Read the model definition and answer for the solid it produces. Units are mm, in the model's axes. A direction names the side the tool comes from. Coordinates: 2 decimals unless noted, no trailing zeros. Order: outer loops, then holes, each group sorted by start corner. A loop starts at its lowest first (then second) coordinate and runs counter-clockwise, first axis right, second up. Notation, with made-up numbers: M 10,59 L 16,59 A19 cw 16,93 Z; hole C 34.5,22 d11. An arc over 180 degrees is marked long. Use a Markdown table: item, result. Add a question column.
1) Find section B-B on y = 10. Write down the section's boundary in (x, z).
2) The mould has two halves that part along X. Classify faces 3 (the face through (1.012, 8.874, 15.317)), 4 (the face through (20.99, 0.493, 16.094)), 5 (the face through (-11, 0, -11)): released by +X, released by -X, zero draft, split by the parting line, or undercut.
3) For faces 1 (the face through (-5, 3, -20)), 2 (the face through (10.15, 1.479, 17.756)), determine the directions among +Z, -Z, +X, -X, +Y, -Y from which every point of the face is accessible in a straight line to the end or side of a thin tool.
4) Find section C-C on y = 4. Write down the section's boundary in (x, z), plus the area to 3 significant figures.
5) Find the intervals of material crossed by probe 1 along Z at (x, y) = (0, 8.75); probe 2 along Y at (x, z) = (22, 7.5); probe 3 along Z at (x, y) = (-22.45, 0.85), in increasing order. Write a range as [from, to].
6) Each of these flat-tipped pins is pushed along its axis until it touches: pin 1 Ø10 at (x, y) = (5.5, 14.5) entering from -Z; pin 2 Ø3.5 at (x, z) = (11.22, -19.44) entering from +Y (3 decimals); pin 3 Ø2 at (y, z) = (10, -1.5) entering from -X; pin 4 Ø5 at (x, z) = (11.22, 19.44) entering from +Y. Where does it stop, or does it pass through?
Autodesk Inventor part; units mm, degrees
ref_plane "YZ Plane" through (0, 0, 0) normal (1, 0, 0) x (0, 1, 0)
ref_plane "XZ Plane" through (0, 0, 0) normal (0, 1, 0) x (-1, 0, 0)
ref_plane "XY Plane" through (0, 0, 0) normal (0, 0, 1) x (1, 0, 0)
sketch "Sketch1" plane through (0, 0, 0) normal (0, 1, 0) x (-1, 0, 0)
  circle A0 centre (0, 0) radius 26.45
  circle A1 centre (22.45, 0) radius 2
  circle A2 centre (0, 0) radius 22.45 construction
  circle A3 centre (-11.225, 19.4423) radius 2
  circle A4 centre (-11.225, -19.4423) radius 2
  circle A5 centre (0, 0) radius 15.35
  dimension "d0" = 52.9
  dimension "d1" = 4
  dimension "d2" = 4
  dimension "d5" = 360
  dimension "d7" = 30.7
extrude "Extrusion1" add sketch "Sketch1" along normal blind 3
sketch "Sketch2" plane through (0, 3, 0) normal (0, 1, 0) x (1, 0, 0)
  circle A0 centre (0, 0) radius 15.35
  circle A1 centre (11.225, 19.4423) radius 2
  circle A2 centre (11.225, -19.4423) radius 2
  circle A3 centre (-22.45, 0) radius 2
  circle A4 centre (0, 0) radius 26.45
  circle A5 centre (0, 0) radius 18.35
  dimension "d10" = 3
extrude "Extrusion2" add sketch "Sketch2" along normal blind 15 contours A5
fillet "Fillet1" radius 2 2 edges at (-18.35, 3, 0) (26.45, 3, 0)
properties part number "00_Zeiss_eyepieceport"
Check result:
| question | item | result |
|---|---|---|
| 1 | outline | C 0,0 d36.7; hole C 0,0 d30.7 |
| 2 | face 3 | undercut |
| 2 | face 4 | split by the parting line |
| 2 | face 5 | zero draft |
| 3 | face 1 | +Y |
| 3 | face 2 | +Y, -Y |
| 4 | outline | C 0,0 d37.24; hole C 0,0 d30.7 |
| 4 | area | 349 mm2 |
| 5 | probe 1 | z = [-18.35, -15.35], [15.35, 18.35] |
| 5 | probe 2 | y = [0, 3] |
| 5 | probe 3 | z = [-13.99, -2], [2, 13.99] |
| 6 | pin 1 | stops at z = -18.34 |
| 6 | pin 2 | passes through |
| 6 | pin 3 | stops at x = -18.34 |
| 6 | pin 4 | stops at y = 3.04 |
